Can you work these out from the model? Positions are in its coordinate system, mm. A direction names the side the tool comes from. Coordinates: 2 decimals unless noted, no trailing zeros. Write each loop counter-clockwise with the first axis right and the second up, starting at its lowest first coordinate (ties: lowest second). Pieces come first, ordered by that corner, then holes. Notation, with made-up numbers: (22.5, 63) - (68.5, 63) arc R20 cw to (68.5, 86) - close; hole circle Ø4 at (76, 51). An arc over 180 degrees is marked (long way). Use one line per item in the form item = value. Start each with the question number.
(1) If we section it at D-D on z = 56.5: Please give me the cut outline in (x, y), then the cut area to 3 significant figures.
(2) For pin 1 Ø3 at (x, y) = (7, -10.5) entering from +Z; pin 2 Ø2.5 at (y, z) = (-64, 18.35) entering from +X; pin 3 Ø1.5 at (x, z) = (8, -54.5) entering from -Y; pin 4 Ø5 at (x, y) = (7, 12) entering from +Z, each with a flat end and sliding along its axis, tell me the tip position at first contact or that it passes through.
(3) If I drill on probe 1 along Z at (x, y) = (9, 0); probe 2 along Z at (x, y) = (1.75, 7); probe 3 along Y at (x, z) = (1, -19.5), over which ranges is the centre line in solid material (lowest first)? Write a range as from..to.
(4) If we section it at C-C on y = -43: Please give me the cut outline in (x, z), then the cut area to 3 significant figures.
(5) If we section it at B-B on z = 77.5: Please give me the cut outline in (x, y).
(6) Thinking about a two-plate mould opening in Y: for faces 1 (the face through (8.028, -66.573, 17.015)), 2 (the face through (5, -67.5, -1)), 3 (the face through (5, 22.5, 1)), which applies, pulls with the +Y half, pulls with the -Y half, needs draft (parallel to the pull), parting line crosses it, or undercut?
(7) If we section it at A-A on y = -19: Please give me the cut outline in (x, z), then the cut area to 3 significant figures.
(8) On a 3-axis mill with a long thin cutter (end or side, diameter ignored), from which of +Z, -Z, +X, -X, +Y, -Y can I reach the whole of each face in a straight line? I mean faces 4 (the face through (5, -1.844, 0)), 5 (the face through (2.51, -9.47, 75.4)), 6 (the face through (8.03, 17.24, -16.05)). Say none if no direction works.
Autodesk Inventor part; units mm, degrees
ref_plane "YZ Plane" through (0, 0, 0) normal (1, 0, 0) x (0, 1, 0)
ref_plane "XZ Plane" through (0, 0, 0) normal (0, 1, 0) x (-1, 0, 0)
ref_plane "XY Plane" through (0, 0, 0) normal (0, 0, 1) x (1, 0, 0)
sketch "Sketch1" plane through (0, 0, 0) normal (1, 0, 0) x (0, 1, 0)
  line L0 (-67.5, 145) -> (67.5, 145)
  line L1 (67.5, 145) -> (67.5, -145)
  line L2 (67.5, -145) -> (-67.5, -145)
  line L3 (-67.5, -145) -> (-67.5, 145)
  line L4 (-67.5, 145) -> (67.5, -145) construction
  line L5 (67.5, 145) -> (-67.5, -145) construction
  circle A0 centre (0, 77.5) radius 5.3
  circle A1 centre (0, -77.5) radius 5.3
  circle A2 centre (0, 0) radius 5.3
  line L6 (0, 77.5) -> (0, -77.5) construction
  line L7 (57.5, -135) -> (57.5, 135)
  line L8 (57.5, 135) -> (-57.5, 135)
  line L9 (-57.5, 135) -> (-57.5, -135)
  line L10 (-57.5, -135) -> (57.5, -135)
  dimension "d0" = 155
  dimension "d1" = 10.6
  dimension "d2" = 290
  dimension "d3" = 135
  dimension "d4" = 10
extrude "Extrusion1" add sketch "Sketch1" along normal blind 10 contours L0 L1 L2 L3 | A2 | L10 L9 L8 L7
chamfer "Chamfer2" distance 20 angle 45 4 edges at (5, 67.5, -145) (5, -67.5, -145) (5, -67.5, 145) (5, 67.5, 145)
sketch "Sketch5" plane through (10, 0, 0) normal (1, 0, 0) x (0, 0, -1)
  line L0 (50, -67.5) -> (-50, -67.5)
  circle A0 centre (0, -15) radius 11
  circle A1 centre (33.234, -33.234) radius 2.75
  circle A2 centre (-33.234, -33.234) radius 2.75
  line L1 (96.4912, -1.1036) -> (50, -67.5)
  line L2 (-50, -67.5) -> (-96.4912, -1.1036)
  arc A3 (-84.2039, 22.5) -> (-96.4912, -1.1036) centre (-84.2039, 7.5) ccw
  line L3 (-84.2039, 22.5) -> (84.2039, 22.5)
  arc A4 (96.4912, -1.1036) -> (84.2039, 22.5) centre (84.2039, 7.5) ccw
  circle A5 centre (-18.3535, 19) radius 1.5
  circle A6 centre (18.3535, -64) radius 1.5
  circle A7 centre (18.3535, 19) radius 1.5
  circle A8 centre (-18.3535, -64) radius 1.5
  point P0 (0, 0)
extrude "Extrusion4" [suppressed]
sketch "Sketch6" plane through (10, 0, 0) normal (1, 0, 0) x (0, 0, -1)
  line L0 (-145, 47.5) -> (-125, 67.5)
  line L1 (-145, 47.5) -> (-145, -47.5)
  line L2 (-125, -67.5) -> (-145, -47.5)
  line L3 (-125, -67.5) -> (125, -67.5)
  line L4 (145, -47.5) -> (125, -67.5)
  line L5 (145, -47.5) -> (145, 47.5)
  line L6 (125, 67.5) -> (145, 47.5)
  line L7 (125, 67.5) -> (-125, 67.5)
  circle A0 centre (-77.5, 0) radius 5.3
  circle A1 centre (77.5, 0) radius 5.3
  circle A2 centre (-131.5, 54) radius 2.9
  circle A3 centre (-96.5, -41.5) radius 2.9
  circle A4 centre (96.5, -41.5) radius 2.9
  circle A5 centre (111.5, 46.5) radius 2.9
  point P0 (0, 0)
  dimension "d21" = 5.8
extrude "Extrusion5" cut sketch "Sketch6" against normal blind 3.5 contours A2 | A3 | A4 | A5
sketch "Sketch7" plane through (10, 0, 0) normal (1, 0, 0) x (0, 0, -1)
  circle A0 centre (96.5, -41.5) radius 2.9
  circle A1 centre (-96.5, -41.5) radius 2.9
  circle A2 centre (111.5, 46.5) radius 2.9
  circle A3 centre (-131.5, 54) radius 2.9
  line L0 (-145, 47.5) -> (-125, 67.5)
  line L1 (-145, 47.5) -> (-145, -47.5)
  line L2 (-125, -67.5) -> (-145, -47.5)
  line L3 (-125, -67.5) -> (125, -67.5)
  line L4 (145, -47.5) -> (125, -67.5)
  line L5 (145, -47.5) -> (145, 47.5)
  line L6 (125, 67.5) -> (145, 47.5)
  line L7 (125, 67.5) -> (-125, 67.5)
  circle A4 centre (-77.5, 0) radius 5.3
  circle A5 centre (77.5, 0) radius 5.3
  line L8 (0, -67.5) -> (0, 22.5)
  line L9 (0, 22.5) -> (-84.2039, 22.5)
  line L10 (-96.4912, -1.1036) -> (-50, -67.5)
  line L11 (-125, -67.5) -> (125, -67.5)
  arc A6 (-84.2039, 22.5) -> (-96.4912, -1.1036) centre (-84.2039, 7.5) ccw
  line L12 (0, 22.5) -> (84.2039, 22.5)
  line L13 (96.4912, -1.1036) -> (50, -67.5)
  arc A7 (96.4912, -1.1036) -> (84.2039, 22.5) centre (84.2039, 7.5) ccw
  point P0 (0, 0)
  point P1 (-50, -67.5)
  point P2 (50, -67.5)
  dimension "d27" = 90
  dimension "d28" = 15
  dimension "d29" = 50
  dimension "d30" = 55
extrude "Extrusion6" cut sketch "Sketch7" against normal through all contours A0 | A1 | A2 | A3 | L0 L7 L6 L5 L4 L3 L13 A7 L12 L9 A6 L10 L2 L1
sketch "Sketch8" plane through (10, 0, 0) normal (1, 0, 0) x (0, 0, -1)
  circle A0 centre (-18.3535, 19) radius 1.5
  circle A1 centre (18.3535, 19) radius 1.5
  circle A2 centre (18.3535, -64) radius 1.5
  circle A3 centre (-18.3535, -64) radius 1.5
  point P0 (0, 0)
extrude "Extrusion7" cut sketch "Sketch8" against normal through all
sketch "Sketch9" plane through (10, 0, 0) normal (1, 0, 0) x (0, 0, -1)
  circle A0 centre (-18.3535, -64) radius 1.5
  circle A1 centre (18.3535, 19) radius 1.5
  circle A2 centre (18.3535, -64) radius 1.5
  circle A3 centre (-18.3535, 19) radius 1.5
  line L0 (-96.4912, -1.1036) -> (-50, -67.5)
  line L1 (-50, -67.5) -> (50, -67.5)
  line L2 (50, -67.5) -> (96.4912, -1.1036)
  arc A4 (96.4912, -1.1036) -> (84.2039, 22.5) centre (84.2039, 7.5) ccw
  line L3 (84.2039, 22.5) -> (-84.2039, 22.5)
  arc A5 (-84.2039, 22.5) -> (-96.4912, -1.1036) centre (-84.2039, 7.5) ccw
  circle A6 centre (-77.5, 0) radius 5.3
  circle A7 centre (77.5, 0) radius 5.3
  circle A8 centre (-18.3535, 19) radius 2.9
  circle A9 centre (18.3535, 19) radius 2.9
  circle A10 centre (-18.3535, -64) radius 2.9
  circle A11 centre (18.3535, -64) radius 2.9
  point P0 (0, 0)
  dimension "d35" = 5.8
extrude "Extrusion8" cut sketch "Sketch9" against normal blind 4 contours A0 | A1 | A2 | A3 | A8 | A9 | A10 | A11
sketch "Sketch10" plane through (10, 0, 0) normal (1, 0, 0) x (0, 0, -1)
  line L0 (-20.1493, -45.8848) -> (20.1493, -45.8848)
  line L1 (30.1493, -35.8848) -> (30.1493, -11.8439)
  line L2 (20.1493, -1.8439) -> (-20.1493, -1.8439)
  line L3 (-30.1493, -11.8439) -> (-30.1493, -35.8848)
  line L4 (-30.1493, -45.8848) -> (30.1493, -1.8439) construction
  line L5 (30.1493, -45.8848) -> (-30.1493, -1.8439) construction
  arc A0 (-20.1493, -1.8439) -> (-30.1493, -11.8439) centre (-20.1493, -11.8439) ccw
  arc A1 (30.1493, -11.8439) -> (20.1493, -1.8439) centre (20.1493, -11.8439) ccw
  arc A2 (20.1493, -45.8848) -> (30.1493, -35.8848) centre (20.1493, -35.8848) ccw
  arc A3 (-30.1493, -35.8848) -> (-20.1493, -45.8848) centre (-20.1493, -35.8848) ccw
  point P0 (0, 0)
  point P1 (0, -23.8644)
  dimension "d38" = 10
extrude "Extrusion9" cut sketch "Sketch10" against normal through all
sketch "Sketch11" plane through (0, 0, 0) normal (-1, 0, 0) x (0, 0, 1)
  circle A0 centre (-77.5, 0) radius 5.3
  circle A1 centre (77.5, 0) radius 5.3
  circle A2 centre (-77.5, 0) radius 9.7
  circle A3 centre (77.5, 0) radius 9.7
  point P0 (0, 0)
  dimension "d41" = 19.4
extrude "Extrusion10" cut sketch "Sketch11" against normal blind 5.1 contours A0 | A1 | A2 | A3
properties part number "CAJA" material "Steel, Mild, Welded"
Reported:
q1.outline = (0, -58.22) - (10, -58.22) - (10, 22.5) - (0, 22.5) - close
q1.area = 807 mm2
q2.pin_1 = 90.96
q2.pin_2 = through
q2.pin_3 = -62.14
q2.pin_4 = 99.07
q3.probe_1 = -97.19..-82.8, -72.2..72.2, 82.8..97.19
q3.probe_2 = -99.2..-84.21, -70.79..70.79, 84.21..99.2
q3.probe_3 = -67.5..-64.97, -63.03..-45.88, -1.84..18.03, 19.97..22.5
q4.outline = (0, -67.16) - (10, -67.16) - (10, -27.18) - (0, -27.18) - close; (0, 27.18) - (10, 27.18) - (10, 67.16) - (0, 67.16) - close
q4.area = 800 mm2
q5.outline = (0, -28.23) - (10, -28.23) - (10, -5.3) - (5.1, -5.3) - (5.1, -9.7) - (0, -9.7) - close; (0, 9.7) - (5.1, 9.7) - (5.1, 5.3) - (10, 5.3) - (10, 22.5) - (0, 22.5) - close
q6.face_1 = undercut
q6.face_2 = pulls with the -Y half
q6.face_3 = pulls with the +Y half
q7.outline = (0, -83.96) - (10, -83.96) - (10, -30.15) - (0, -30.15) - close; (0, 30.15) - (10, 30.15) - (10, 83.96) - (0, 83.96) - close
q7.area = 1,080 mm2
q8.face_4 = +X, -X
q8.face_5 = -X
q8.face_6 = +X
